from build123d import *

# Parameters (mm, degrees)
SKETCH_W        = 263.525
SKETCH_H        = 117.475
PAD_DEPTH       = 3.175
SKETCH002_W     = 249.2375
SKETCH002_H     = 77.7875
POCKET_DEPTH    = 3.176
SKETCH003_R     = 7.5
POCKET001_DEPTH = 3.176
SKETCH001_R     = 1.05029
HOLE_DEPTH      = 3.176
FILLET_R        = 5.08
FILLET001_R     = 1.27


with BuildPart() as part:
    # Sketch → Pad (new body)
    with BuildSketch(Plane.XY):
        Rectangle(SKETCH_W, SKETCH_H)
    extrude(amount=PAD_DEPTH)

    # Sketch002 (on Face6 of Pad) → Pocket (cut, through all)
    with BuildSketch(Plane.XY.offset(3.175)):
        with Locations((0, -12.7)):
            Rectangle(SKETCH002_W, SKETCH002_H)
    extrude(amount=-POCKET_DEPTH, mode=Mode.SUBTRACT)

    # Sketch003 (on Face5 of Pocket) → Pocket001 (cut, through all)
    with BuildSketch(Plane.XY.offset(3.175)):
        with Locations((98.425, 39.37)):
            Circle(SKETCH003_R)
    extrude(amount=-POCKET001_DEPTH, mode=Mode.SUBTRACT)

    # Sketch001 (on Face6 of Pad) → Hole (cut, through all)
    with BuildSketch(Plane.XY.offset(3.175)):
        with Locations((-42.597917, 54.76875)):
            Circle(SKETCH001_R)
        with Locations((42.597917, 54.76875)):
            Circle(SKETCH001_R)
        with Locations((42.597917, -54.76875)):
            Circle(SKETCH001_R)
        with Locations((-42.597917, -54.76875)):
            Circle(SKETCH001_R)
        with Locations((-127.79375, -54.76875)):
            Circle(SKETCH001_R)
        with Locations((-127.79375, 54.76875)):
            Circle(SKETCH001_R)
        with Locations((127.79375, 54.76875)):
            Circle(SKETCH001_R)
        with Locations((127.79375, -54.76875)):
            Circle(SKETCH001_R)
    extrude(amount=-HOLE_DEPTH, mode=Mode.SUBTRACT)

    # Fillet
    fillet_edges = [part.edges().sort_by_distance(p)[0] for p in [
        (-131.7625, 58.7375, 1.5875),
        (-131.7625, -58.7375, 1.5875),
        (131.7625, -58.7375, 1.5875),
        (131.7625, 58.7375, 1.5875),
    ]]
    fillet(fillet_edges, radius=FILLET_R)

    # Fillet001
    fillet001_edges = [part.edges().sort_by_distance(p)[0] for p in [
        (-124.61875, -51.59375, 1.5875),
        (-124.61875, 26.19375, 1.5875),
        (124.61875, 26.19375, 1.5875),
        (124.61875, -51.59375, 1.5875),
    ]]
    fillet(fillet001_edges, radius=FILLET001_R)


solid = part.part
Source: CAD feature listing. Evaluate the final solid. Frame: model axes, mm. Round coordinates to 2 decimals unless told otherwise and drop trailing zeros. Order: outer loops, then holes, each group sorted by start corner. A loop starts at its lowest first (then second) coordinate and runs counter-clockwise, first axis right, second up. Notation, with made-up numbers: (11.5, 46) - (39.5, 46) arc R35 cw to (39.5, 85) - close; hole circle Ø10 at (73.25, 84). An arc over 180 degrees is marked (long way). Use a Markdown table: item, result. Add a question column.
1. Section query D-D (x = 95). Return the cut outline in (y, z) (1 decimal), then the cut area to 3 significant figures.
2. Line query: probe 1 along Y at (x, z) = (26.5, 1.55); probe 2 along X at (y, z) = (5.5, 3); probe 3 along X at (y, z) = (39.5, 3). Output: solid intervals per line, ascending.
3. Mould query, pull axis X, two halves, no side actions, for faces 1 (the flat face through (-1, 35, 3.175)), 2 (the cylindrical face through (105.58, 41.62, 1.61)), 3 (the cylindrical face through (130.235, 57.289, 1.61)). Classes: +X half, -X half, draft (parallel to the pull), parting line (faces both ways), or undercut.
4. Section query A-A (y = 39.37). Return the cut outline in (x, z) (1 decimal).
5. First-contact query: pin 1 (3.5 mm diameter, centred on x = 127.79, y = 54.77, fed in from +Z) (3 decimals); pin 2 (1.7 mm diameter, centred on x = -127.79, y = 54.77, fed in from +Z). Flat tips, straight axial feed; report the tip coordinate or a pass-through.
6. Section query C-C (z = 1.05). Give the number of separate pieces and of enclosed holes in the cut face, then the cut area to 3 significant figures.
7. Section query B-B (x = -15.5). Return the cut outline in (y, z) (1 decimal).
Derived:
| question | item | result |
|---|---|---|
| 1 | outline | (-58.7, 0) - (-51.6, 0) - (-51.6, 3.2) - (-58.7, 3.2) - close; (26.2, 0) - (32.7, 0) - (32.7, 3.2) - (26.2, 3.2) - close; (46, 0) - (58.7, 0) - (58.7, 3.2) - (46, 3.2) - close |
| 1 | area | 83.6 mm2 |
| 2 | probe 1 | -58.74 to -51.59, 26.19 to 58.74 |
| 2 | probe 2 | -131.76 to -124.62, 124.62 to 131.76 |
| 2 | probe 3 | -131.76 to 90.93, 105.92 to 131.76 |
| 3 | face 1 | draft |
| 3 | face 2 | undercut |
| 3 | face 3 | +X half |
| 4 | outline | (-131.8, 0) - (90.9, 0) - (90.9, 3.2) - (-131.8, 3.2) - close; (105.9, 0) - (131.8, 0) - (131.8, 3.2) - (105.9, 3.2) - close |
| 5 | pin 1 | z = 3.175 |
| 5 | pin 2 | through |
| 6 | separate pieces | 1 |
| 6 | enclosed holes | 10 |
| 6 | area | 11,300 mm2 |
| 7 | outline | (-58.7, 0) - (-51.6, 0) - (-51.6, 3.2) - (-58.7, 3.2) - close; (26.2, 0) - (58.7, 0) - (58.7, 3.2) - (26.2, 3.2) - close |
